```python
from build123d import *

# Parameters (mm, degrees)
F0_W     = 18
F0_H     = 18
F1_DEPTH = 100
F3_D     = 6.8
F5_D     = 3.3
F5_DEPTH = 8
F5_TIP   = 0.9914200214
F8_D     = 5
F8_DEPTH = 18
F8_TIP   = 1.5021515476
F7_W     = 18
F7_H     = 18
F9_DEPTH = 9


with BuildPart() as f1:
    # F0 (on Right) → F1 (new body, symmetric)
    with BuildSketch(Plane.YZ):
        with Locations((-3.1000529416, 1.3550933172)):
            Rectangle(F0_W, F0_H)
    extrude(amount=F1_DEPTH, both=True)

    # F3 (through all)
    with Locations(Plane.XY.offset(10.3550933172)):
        with Locations((-10, -3.1000529416), (10, -3.1000529416)):
            Hole(F3_D / 2)

    # F5
    with Locations(Plane(origin=(0, 5.8999470584, 0), x_dir=(-1, 0, 0), z_dir=(0, 1, 0))):
        with Locations((-10, 2.3550933172), (10, 2.3550933172)):
            Hole(F5_D / 2, depth=F5_DEPTH)
            with Locations((0, 0, -(F5_DEPTH + F5_TIP / 2))):  # 118° drill point
                Cone(0, F5_D / 2, F5_TIP, mode=Mode.SUBTRACT)

    # F8
    with Locations(Plane(origin=(0, 0, -7.6449066828), x_dir=(1, 0, 0), z_dir=(0, 0, -1))):
        with Locations((91, 3.1000529416), (-91, 3.1000529416)):
            Hole(F8_D / 2, depth=F8_DEPTH)
            with Locations((0, 0, -(F8_DEPTH + F8_TIP / 2))):  # 118° drill point
                Cone(0, F8_D / 2, F8_TIP, mode=Mode.SUBTRACT)

    # F7 (on face) → F9 (cut)
    with BuildSketch(Plane(origin=(0, 0, -7.6449066828), x_dir=(1, 0, 0), z_dir=(0, 0, -1))):
        with Locations((-91, 3.1000529416)):
            Rectangle(F7_W, F7_H)
        with Locations((91, 3.1000529416)):
            Rectangle(F7_W, F7_H)
    extrude(amount=-F9_DEPTH, mode=Mode.SUBTRACT)


solid = f1.part
```
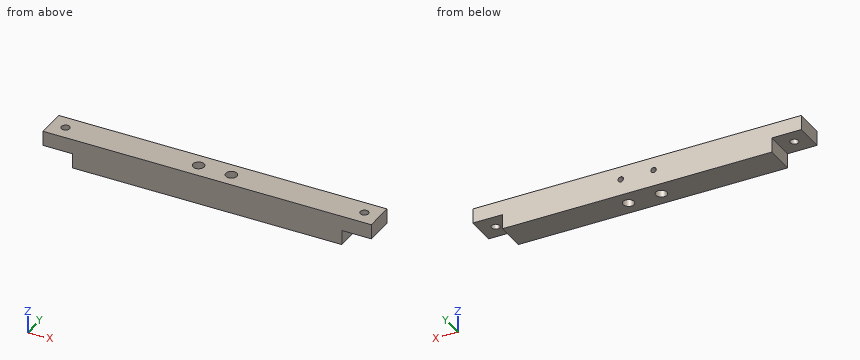
Build history of the part. All positions in model axes, mm. Round coordinates to 2 decimals unless told otherwise and drop trailing zeros. Loops run counter-clockwise (first coordinate to the right, second up) from the corner with the lowest first, then second, coordinate; pieces in that order, holes last. Notation, with made-up numbers: M -30.75,64 L -13.75,64 A36 ccw -13.75,101 Z; hole C 82.5,-39 d5. An arc over 180 degrees is marked long. Answer as CSV lines item,"result".
1. Wall check: probe 1 along X at (y, z) = (-3, 5.5); probe 2 along X at (y, z) = (-1.75, 9); probe 3 along X at (y, z) = (-1.75, -0.5). Give the ranges that are in metal, low to high. Write a range as [from, to].
Resolved:
probe 1,"x = [-100, -93.5], [-88.5, -13.4], [-6.6, 6.6], [13.4, 88.5], [93.5, 100]"
probe 2,"x = [-100, -93.1], [-88.9, -13.12], [-6.88, 6.88], [13.12, 88.9], [93.1, 100]"
probe 3,"x = [-82, -13.12], [-6.88, 6.88], [13.12, 82]"
2. Cut at C-C on y = -8.25. Write the cut outline in (x, z).
Resolved:
outline,"M -100,1.36 L -82,1.36 L -82,-7.64 L 82,-7.64 L 82,1.36 L 100,1.36 L 100,10.36 L -100,10.36 Z"
3. Flat gauge pins, fed straight in: P1, Ø3, axis at y = -8.5, z = -4, coming from the -X side; P2, Ø9, axis at x = 94.5, y = -5.5, coming from the -Z side; P3, Ø2.5, axis at y = -3.5, z = -5, coming from the +X side. Where does each tip first touch, or does it go through?
Resolved:
P1,"stops at x = -82"
P2,"stops at z = 1.36"
P3,"stops at x = 82"
4. Cut at A-A on x = -91. Write the cut outline in (y, z), then the cut area to 3 significant figures.
Resolved:
outline,"M -12.1,1.36 L -5.6,1.36 L -5.6,10.36 L -12.1,10.36 Z; M -0.6,1.36 L 5.9,1.36 L 5.9,10.36 L -0.6,10.36 Z"
area,"117 mm²"
5. Cut at D-D on z = -4.5. Write the cut outline in (x, y).
Resolved:
outline,"M -82,-12.1 L 82,-12.1 L 82,5.9 L -82,5.9 Z; hole C -10,-3.1 d6.8; hole C 10,-3.1 d6.8"
6. Cut at B-B on x = 10. Write the cut outline in (y, z).
Resolved:
outline,"M -12.1,-7.64 L -6.5,-7.64 L -6.5,10.36 L -12.1,10.36 Z; M 0.3,-7.64 L 5.9,-7.64 L 5.9,0.71 L 0.3,0.71 Z; M 0.3,4.01 L 5.9,4.01 L 5.9,10.36 L 0.3,10.36 Z"
